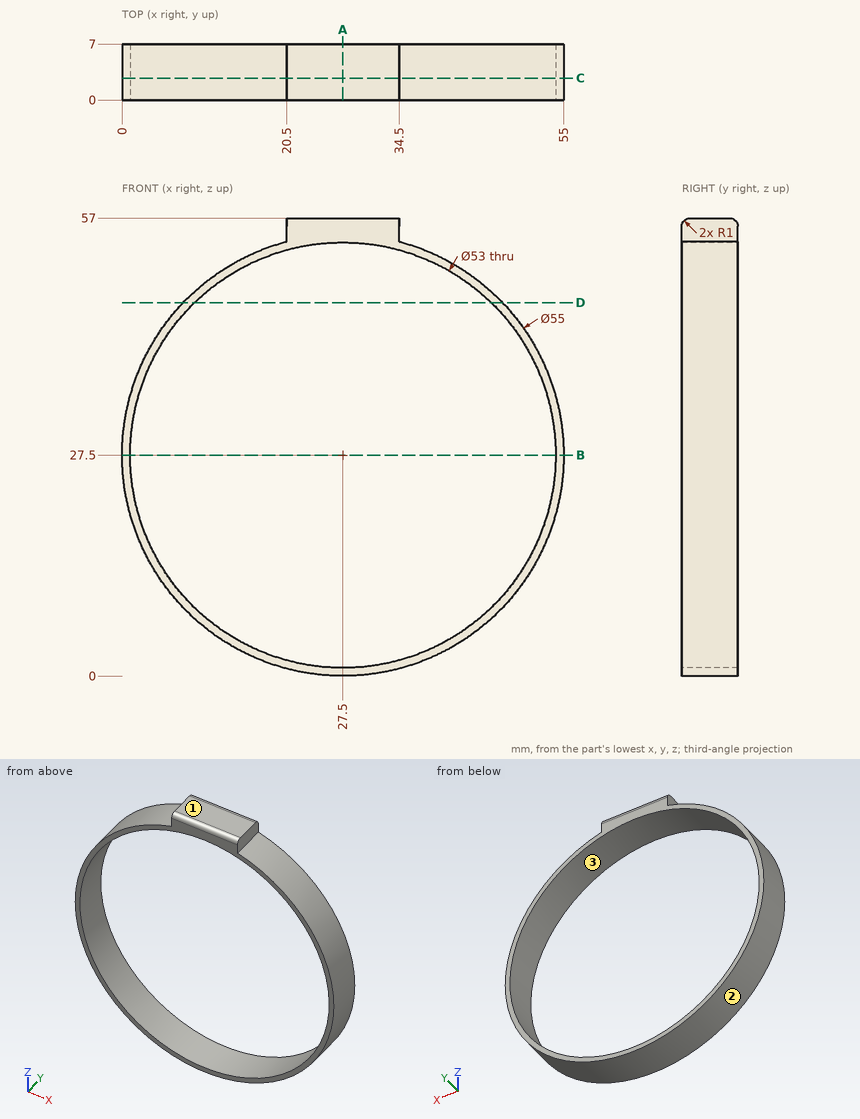
Part print with two shaded views. Sizes in mm from the minimum x, y, z corner. Give positions to 0.01 mm unless a question says otherwise; leave off trailing zeros. Order: outer loops, then holes, each group sorted by start corner. A loop starts at its lowest first (then second) coordinate and runs counter-clockwise, first axis right, second up. Notation, with made-up numbers: (41, 80.5) - (92, 80.5) arc R26 cw to (92, 107.5) - close; hole circle Ø4 at (49.25, -10). An arc over 180 degrees is marked (long way). Write each question's results on one line, items separated by ' | '.
1. Pull direction Z, two halves, no side cores. Call the marked faces 1, 2 and 3: released by +Z, released by -Z, zero draft, split by the parting line, or undercut.
Calculated:
face 1: released by +Z | face 2: split by the parting line | face 3: undercut
2. Probe L1, parallel to X at y = 5.5, z = 27.5; L2, parallel to Z at x = 50.5, y = 5; L3, parallel to X at y = 4.75, z = 4. List the from-to ranges inside material, lowest first. Write a range as from..to.
Calculated:
L1: x = 0..1, 54..55 | L2: z = 12.43..14.34, 40.66..42.57 | L3: x = 13.22..15.25, 39.75..41.78
3. Saw through at A-A on x = 27.5. List the corners of the cut face in (y, z).
Calculated:
outline: (0, 0) - (7, 0) - (7, 1) - (0, 1) - close; (0, 54) - (7, 54) - (7, 56) arc R1 ccw to (6, 57) - (1, 57) arc R1 ccw to (0, 56) - close
4. Pin check, flat tips, straight feed: pin 1 (4 mm diameter, centred on x = 29.5, y = 1, fed in from -Z); pin 2 (1.5 mm diameter, centred on y = 4.5, z = 55.5, fed in from +X); pin 3 (4 mm diameter, centred on y = 1.5, z = 32, fed in from +X). Stop position of each tip, or through.
Calculated:
pin 1: stops at z = 0 | pin 2: stops at x = 34.5 | pin 3: stops at x = 54.89
5. Saw through at D-D on z = 46.5. List the corners of the cut face in (x, y).
Calculated:
outline: (7.62, 0) - (9.03, 0) - (9.03, 7) - (7.62, 7) - close; (45.97, 0) - (47.38, 0) - (47.38, 7) - (45.97, 7) - close
6. Saw through at C-C on y = 2.75. List the corners of the cut face in (x, z), and give its area (3 significant figures).
Calculated:
outline: (20.5, 54.09) arc R27.5 ccw (long way) to (34.5, 54.09) - (34.5, 57) - (20.5, 57) - close; hole circle Ø53 at (27.5, 27.5) | area: 202 mm2
7. Saw through at B-B on z = 27.5. List the corners of the cut face in (x, y).
Calculated:
outline: (0, 0) - (1, 0) - (1, 7) - (0, 7) - close; (54, 0) - (55, 0) - (55, 7) - (54, 7) - close
